Part model, mm, in its own coordinate system. A direction names the side the tool comes from. Round coordinates to 2 decimals unless told otherwise and drop trailing zeros. Write each loop counter-clockwise with the first axis right and the second up, starting at its lowest first coordinate (ties: lowest second). Pieces come first, ordered by that corner, then holes. Notation, with made-up numbers: M 71,78 L 85,78 A18 cw 85,94 Z; hole C 4.25,4 d11. An arc over 180 degrees is marked long. Answer as a JSON object with one key per item and string values. Group by question number.
1. Drill centre lines: line 1 (X direction, y = 19.5, z = 0.6); line 2 (X direction, y = 20, z = 2.35); line 3 (Z direction, x = 14.5, y = 24). Where is each one in solid material? Low to high. Write a range as from..to.
2. Which spindle directions (+Z, -Z, +X, -X, +Y, -Y) get a long thin tool onto all of the face, cutting with end or side? Do faces 1 (the face through (19, 15, 1)), 2 (the face through (19, 38, 1)). Say none if no direction does.
3. Band-saw the part on D-D, the plane y = 27. Write the cut outline in (x, z), plus the area to 3 significant figures.
4. Drop flat-ended pins along their axis: pin 1 (0.7 mm diameter, centred on x = 16.5, z = 2.5, fed in from -Y); pin 2 (0.5 mm diameter, centred on x = 33, z = 2, fed in from +Y); pin 3 (1.5 mm diameter, centred on x = 4, y = 9, fed in from +Z). Give the stop position or say it passes through.
5. Band-saw the part on C-C, the plane z = 0.95. Write the cut outline in (x, y), plus the area to 3 significant figures.
6. Two-plate mould, pull along Y, no slides. Class faces 3 (the face through (33, 19, 2.6)), 4 (the face through (35.861, 35.745, 1.014)), 5 (the face through (19, 23, 1)): +Y half, -Y half, draft (parallel to the pull), parting line (faces both ways), or undercut.
7. Band-saw the part on A-A, the plane y = 22. Write the cut outline in (x, z), plus the area to 3 significant figures.
Autodesk Fusion 360 part; units mm, degrees
sketch "Sketch1" plane through (0, 0, 0) normal (0, 0, 1) x (1, 0, 0)
  line L0 (0, 0) -> (38, 0)
  line L1 (38, 0) -> (38, 38)
  line L2 (38, 38) -> (0, 38)
  line L3 (0, 38) -> (0, 0)
  dimension "d1" = 38
  dimension "d2" = 38
extrude "Extrude1" add sketch "Sketch1" along normal blind 2
sketch "Sketch2" plane through (0, 0, 2) normal (0, 0, 1) x (-1, 0, 0)
  line L0 (0, -38) -> (0, 0)
  line L1 (0, 0) -> (-38, 0)
  line L2 (-38, 0) -> (-38, -38)
  line L3 (-38, -38) -> (0, -38)
  line L4 (-23, -23) -> (-23, -15)
  line L5 (-23, -15) -> (-15, -15)
  line L6 (-15, -15) -> (-15, -23)
  line L7 (-15, -23) -> (-23, -23)
  dimension "d6" = 8
  dimension "d7" = 8
  dimension "d8" = 8
  dimension "d9" = 15
  dimension "d10" = 15
extrude "Extrude2" cut sketch "Sketch2" against normal blind 7 contours L4 L5 L6 L7
sketch "Sketch3" plane through (0, 0, 2) normal (0, 0, 1) x (-1, 0, 0)
  line L0 (-23, -15) -> (-15, -15)
  line L1 (-15, -15) -> (-15, -23)
  line L2 (-15, -23) -> (-23, -23)
  line L3 (-23, -23) -> (-23, -15)
  line L4 (0, -38) -> (0, 0)
  line L5 (0, 0) -> (-38, 0)
  line L6 (-38, 0) -> (-38, -38)
  line L7 (-38, -38) -> (0, -38)
  line L8 (-15, -23) -> (-15, -28)
  line L9 (-15, -28) -> (-10, -28)
  line L10 (-10, -28) -> (-28, -28)
  line L11 (-28, -28) -> (-28, -10)
  line L12 (-28, -10) -> (-10, -10)
  line L13 (-10, -10) -> (-10, -28)
  line L14 (-31, -28) -> (-35, -28)
  line L15 (-35, -28) -> (-35, -10)
  line L16 (-35, -10) -> (-31, -10)
  line L17 (-31, -10) -> (-31, -28)
  line L18 (-19, -28) -> (-19, -10)
  line L19 (-28, -28) -> (-10, -10)
  line L20 (-28, -31) -> (-28, -35)
  line L21 (-10, -31) -> (-28, -31)
  line L22 (-28, -35) -> (-10, -35)
  line L23 (-10, -35) -> (-10, -31)
  line L24 (-7, -10) -> (-7, -28)
  line L25 (-7, -28) -> (-3, -28)
  line L26 (-3, -28) -> (-3, -10)
  line L27 (-3, -10) -> (-7, -10)
  line L28 (-31.1, -27.9) -> (-34.9, -27.9)
  line L29 (-34.9, -27.9) -> (-34.9, -10.1)
  line L30 (-34.9, -10.1) -> (-31.1, -10.1)
  line L31 (-31.1, -10.1) -> (-31.1, -27.9)
  line L32 (-27.9, -31.1) -> (-27.9, -34.9)
  line L33 (-10.1, -31.1) -> (-27.9, -31.1)
  line L34 (-27.9, -34.9) -> (-10.1, -34.9)
  line L35 (-10.1, -34.9) -> (-10.1, -31.1)
  line L36 (-6.9, -27.9) -> (-3.1, -27.9)
  line L37 (-6.9, -10.1) -> (-6.9, -27.9)
  line L38 (-3.1, -27.9) -> (-3.1, -10.1)
  line L39 (-3.1, -10.1) -> (-6.9, -10.1)
  dimension "d13" = 5
  dimension "d14" = 5
  dimension "d15" = 18
  dimension "d16" = 18
  dimension "d17" = 4
  dimension "d18" = 3
  dimension "d19" = 0.1
  dimension "d20" = 0.1
  dimension "d21" = 0.1
  dimension "d22" = 0.1
extrude "Extrude3" add sketch "Sketch3" along normal blind 0.6 contours L28 L29 L30 L31 | L32 L33 L34 L35 | L36 L37 L38 L39
fillet "Fillet1" radius 7.5 2 edges at (0, 38, 1) (38, 38, 1)
chamfer "Chamfer2" distance 2 angle 45 1 edges at (19, 0, 0)
Worked answers:
{
 "1": {"line 1": "x = 0..15, 23..38", "line 2": "x = 3.1..6.9, 31.1..34.9", "line 3": "z = 0..2"},
 "2": {"face 1": "+Z, -Z", "face 2": "+Z, -Z, +X, -X, +Y"},
 "3": {"outline": "M 0,0 L 38,0 L 38,2 L 34.9,2 L 34.9,2.6 L 31.1,2.6 L 31.1,2 L 6.9,2 L 6.9,2.6 L 3.1,2.6 L 3.1,2 L 0,2 Z", "area": "80.6 mm^2"},
 "4": {"pin 1": "stops at y = 31.1", "pin 2": "stops at y = 37.65", "pin 3": "stops at z = 2"},
 "5": {"outline": "M 0,1.05 L 38,1.05 L 38,30.5 A7.5 ccw 30.5,38 L 7.5,38 A7.5 ccw 0,30.5 Z; hole M 15,15 L 23,15 L 23,23 L 15,23 Z", "area": "1,320 mm^2"},
 "6": {"face 3": "draft", "face 4": "+Y half", "face 5": "undercut"},
 "7": {"outline": "M 0,0 L 15,0 L 15,2 L 6.9,2 L 6.9,2.6 L 3.1,2.6 L 3.1,2 L 0,2 Z; M 23,0 L 38,0 L 38,2 L 34.9,2 L 34.9,2.6 L 31.1,2.6 L 31.1,2 L 23,2 Z", "area": "64.6 mm^2"}
}
